```python
from build123d import *

# Parameters (mm, degrees)
ESQUISSE1_R             = 2
BOSS_EXTRU_1_DEPTH      = 3
CONG_2_R                = 10
CONG_3_R                = 10
ENL_V_MAT_EXTRU_1_DEPTH = 198.287332615
CONG_4_R                = 5


with BuildPart() as part:
    # Esquisse1 → Boss.-Extru.1 (new body)
    with BuildSketch(Plane(origin=(0, 0, 0), x_dir=(1, 0, 0), z_dir=(0, 1, 0))):
        Polygon((-150, 0), (-75, -129.903810568), (75, -129.903810568), (150, 0), (75, 129.903810568), (-75, 129.903810568), align=None)
        with Locations(Location((15.5, -109.903810568, 0), (0, 0, 270))):
            Circle(ESQUISSE1_R, mode=Mode.SUBTRACT)
        with Locations(Location((-15.5, -109.903810568, 0), (0, 0, 90))):
            Circle(ESQUISSE1_R, mode=Mode.SUBTRACT)
        with Locations(Location((15.5, -59.903810568, 0), (0, 0, 270))):
            Circle(ESQUISSE1_R, mode=Mode.SUBTRACT)
        with Locations(Location((-15.5, -59.903810568, 0), (0, 0, 90))):
            Circle(ESQUISSE1_R, mode=Mode.SUBTRACT)
        with Locations(Location((-87.429491924, -68.375299042, 0), (0, 0, 270))):
            Circle(ESQUISSE1_R, mode=Mode.SUBTRACT)
        with Locations(Location((-102.929491924, -41.528511525, 0), (0, 0, 90))):
            Circle(ESQUISSE1_R, mode=Mode.SUBTRACT)
        with Locations(Location((-59.628221735, -16.528511525, 0), (0, 0, 90))):
            Circle(ESQUISSE1_R, mode=Mode.SUBTRACT)
        with Locations(Location((-44.128221735, -43.375299042, 0), (0, 0, 270))):
            Circle(ESQUISSE1_R, mode=Mode.SUBTRACT)
        with Locations(Location((-102.929491924, 41.528511525, 0), (0, 0, 270))):
            Circle(ESQUISSE1_R, mode=Mode.SUBTRACT)
        with Locations(Location((-87.429491924, 68.375299042, 0), (0, 0, 90))):
            Circle(ESQUISSE1_R, mode=Mode.SUBTRACT)
        with Locations(Location((-44.128221735, 43.375299042, 0), (0, 0, 90))):
            Circle(ESQUISSE1_R, mode=Mode.SUBTRACT)
        with Locations(Location((-59.628221735, 16.528511525, 0), (0, 0, 270))):
            Circle(ESQUISSE1_R, mode=Mode.SUBTRACT)
        with Locations(Location((-15.5, 109.903810568, 0), (0, 0, 270))):
            Circle(ESQUISSE1_R, mode=Mode.SUBTRACT)
        with Locations(Location((15.5, 109.903810568, 0), (0, 0, 90))):
            Circle(ESQUISSE1_R, mode=Mode.SUBTRACT)
        with Locations(Location((15.5, 59.903810568, 0), (0, 0, 90))):
            Circle(ESQUISSE1_R, mode=Mode.SUBTRACT)
        with Locations(Location((-15.5, 59.903810568, 0), (0, 0, 270))):
            Circle(ESQUISSE1_R, mode=Mode.SUBTRACT)
        with Locations(Location((87.429491924, 68.375299042, 0), (0, 0, 270))):
            Circle(ESQUISSE1_R, mode=Mode.SUBTRACT)
        with Locations(Location((102.929491924, 41.528511525, 0), (0, 0, 90))):
            Circle(ESQUISSE1_R, mode=Mode.SUBTRACT)
        with Locations(Location((59.628221735, 16.528511525, 0), (0, 0, 90))):
            Circle(ESQUISSE1_R, mode=Mode.SUBTRACT)
        with Locations(Location((44.128221735, 43.375299042, 0), (0, 0, 270))):
            Circle(ESQUISSE1_R, mode=Mode.SUBTRACT)
        with Locations(Location((102.929491924, -41.528511525, 0), (0, 0, 270))):
            Circle(ESQUISSE1_R, mode=Mode.SUBTRACT)
        with Locations(Location((87.429491924, -68.375299042, 0), (0, 0, 90))):
            Circle(ESQUISSE1_R, mode=Mode.SUBTRACT)
        with Locations(Location((44.128221735, -43.375299042, 0), (0, 0, 90))):
            Circle(ESQUISSE1_R, mode=Mode.SUBTRACT)
        with Locations(Location((59.628221735, -16.528511525, 0), (0, 0, 270))):
            Circle(ESQUISSE1_R, mode=Mode.SUBTRACT)
    extrude(amount=BOSS_EXTRU_1_DEPTH)

    # Congé2
    cong_2_edges = [part.edges().sort_by_distance(p)[0] for p in [
        (-75, 1.5, -129.903810568),
    ]]
    fillet(cong_2_edges, radius=CONG_2_R)

    # Congé3
    cong_3_edges = [part.edges().sort_by_distance(p)[0] for p in [
        (75, 1.5, -129.903810568),
        (150, 1.5, 0),
        (75, 1.5, 129.903810568),
        (-75, 1.5, 129.903810568),
        (-150, 1.5, 0),
    ]]
    fillet(cong_3_edges, radius=CONG_3_R)

    # Esquisse3 → Enlèv. mat.-Extru.1 (cut, through all)
    with BuildSketch(Plane(origin=(0, 3, 0), x_dir=(1, 0, 0), z_dir=(0, 1, 0))):
        with BuildLine():
            Line((-69.226497308, -129.903810568), (-29.814110868, -129.903810568))
            Line((-29.814110868, -129.903810568), (-29.814110868, -51.639554805))
            Line((-29.814110868, -51.639554805), (-97.592944566, -90.771682686))
            Line((-97.592944566, -90.771682686), (-77.886751346, -124.903810568))
            ThreePointArc((-77.886751346, -124.903810568), (-74.226497308, -128.564064606), (-69.226497308, -129.903810568))
        make_face()
        with BuildLine():
            Line((-147.113248654, -5), (-127.5737221, -38.843452747))
            Line((-127.5737221, -38.843452747), (-59.794888402, 0.288675135))
            Line((-59.794888402, 0.288675135), (-127.0737221, 39.132127881))
            Line((-127.0737221, 39.132127881), (-127.3237221, 39.276465449))
            Line((-127.3237221, 39.276465449), (-147.113248654, 5))
            ThreePointArc((-147.113248654, 5), (-148.452994616, 0), (-147.113248654, -5))
        make_face()
        with BuildLine():
            Line((-77.886751346, 124.903810568), (-97.592944566, 90.771682686))
            Line((-97.592944566, 90.771682686), (-97.092944566, 90.483007552))
            Line((-97.092944566, 90.483007552), (-29.814110868, 51.639554805))
            Line((-29.814110868, 51.639554805), (-29.814110868, 129.903810568))
            Line((-29.814110868, 129.903810568), (-69.226497308, 129.903810568))
            ThreePointArc((-69.226497308, 129.903810568), (-74.226497308, 128.564064606), (-77.886751346, 124.903810568))
        make_face()
        with BuildLine():
            Line((30.147444201, 51.639554805), (97.6762779, 90.627345119))
            Line((97.6762779, 90.627345119), (77.886751346, 124.903810568))
            ThreePointArc((77.886751346, 124.903810568), (74.226497308, 128.564064606), (69.226497308, 129.903810568))
            Line((69.226497308, 129.903810568), (30.147444201, 129.903810568))
            Line((30.147444201, 129.903810568), (30.147444201, 129.326460298))
            Line((30.147444201, 129.326460298), (30.147444201, 51.639554805))
        make_face()
        with BuildLine():
            Line((60.128221735, -0.288675135), (127.407055434, -39.132127881))
            Line((127.407055434, -39.132127881), (147.113248654, -5))
            ThreePointArc((147.113248654, -5), (148.452994616, 0), (147.113248654, 5))
            Line((147.113248654, 5), (127.407055434, 39.132127881))
            Line((127.407055434, 39.132127881), (59.628221735, 0))
            Line((59.628221735, 0), (60.128221735, -0.288675135))
        make_face()
        with BuildLine():
            Line((29.647444201, -51.92822994), (29.647444201, -129.903810568))
            Line((29.647444201, -129.903810568), (69.226497308, -129.903810568))
            ThreePointArc((69.226497308, -129.903810568), (74.226497308, -128.564064606), (77.886751346, -124.903810568))
            Line((77.886751346, -124.903810568), (97.4262779, -91.060357821))
            Line((97.4262779, -91.060357821), (29.647444201, -51.92822994))
        make_face()
        with BuildLine():
            Line((-32.564110868, -20.388611416), (-32.564110868, 22.986687627))
            ThreePointArc((-32.564110868, 22.986687627), (-37.564110868, 27.986687627), (-42.564110868, 22.986687627))
            Line((-42.564110868, 22.986687627), (-42.564110868, -20.388611416))
            ThreePointArc((-42.564110868, -20.388611416), (-37.564110868, -25.388611416), (-32.564110868, -20.388611416))
        make_face()
        with BuildLine():
            Line((33.939110868, -16.708003449), (-3.625, -38.395652971))
            ThreePointArc((-3.625, -38.395652971), (-5.455127019, -45.22577999), (1.375, -47.055907009))
            Line((1.375, -47.055907009), (38.939110868, -25.368257487))
            ThreePointArc((38.939110868, -25.368257487), (40.769237886, -18.538130468), (33.939110868, -16.708003449))
        make_face()
        with BuildLine():
            Line((-2.5, 39.045172024), (35.064110868, 17.357522502))
            ThreePointArc((35.064110868, 17.357522502), (41.894237886, 19.187649521), (40.064110868, 26.01777654))
            Line((40.064110868, 26.01777654), (2.5, 47.705426061))
            ThreePointArc((2.5, 47.705426061), (-4.330127019, 45.875299042), (-2.5, 39.045172024))
        make_face()
    extrude(amount=-ENL_V_MAT_EXTRU_1_DEPTH, mode=Mode.SUBTRACT)

    # Congé4
    cong_4_edges = [part.edges().sort_by_distance(p)[0] for p in [
        (-127.5737221, 1.5, 38.843452747),
        (-127.3237221, 1.5, -39.276465449),
        (-59.794888402, 1.5, -0.288675135),
        (-97.592944566, 1.5, -90.771682686),
        (-29.814110868, 1.5, -129.903810568),
        (-29.814110868, 1.5, -51.639554805),
        (30.147444201, 1.5, -129.903810568),
        (97.6762779, 1.5, -90.627345119),
        (30.147444201, 1.5, -51.639554805),
        (127.407055434, 1.5, -39.132127881),
        (127.407055434, 1.5, 39.132127881),
        (59.628221735, 1.5, 0),
        (97.4262779, 1.5, 91.060357821),
        (29.647444201, 1.5, 129.903810568),
        (29.647444201, 1.5, 51.92822994),
        (-29.814110868, 1.5, 51.639554805),
        (-29.814110868, 1.5, 129.903810568),
        (-97.592944566, 1.5, 90.771682686),
    ]]
    fillet(cong_4_edges, radius=CONG_4_R)


solid = part.part
```
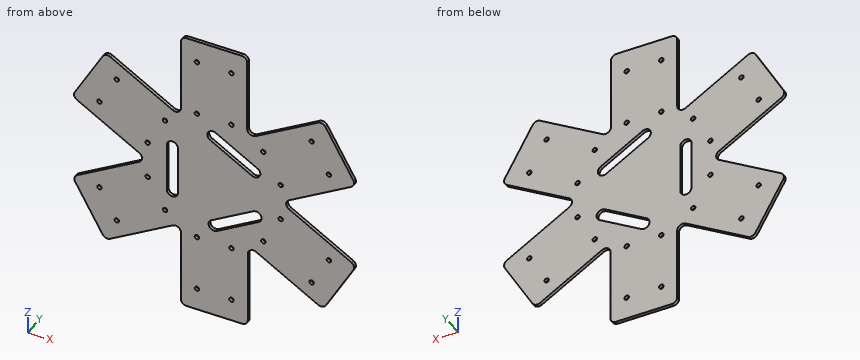
Geometry: final body of the model. Coordinates: model frame, mm. Give positions to 0.01 mm unless a question says otherwise; leave off trailing zeros. Loops run counter-clockwise (first coordinate to the right, second up) from the corner with the lowest first, then second, coordinate; pieces in that order, holes last. Notation, with made-up numbers: (0, 36.5) - (37, 36.5) arc R13 cw to (37, 50.5) - close; hole circle Ø10 at (24, -20). An arc over 180 degrees is marked (long way). Answer as CSV lines item,"result". Start each with the question number.
(1) Ray query, line 1 along Z through (x, y) = (-15, 2.7); line 2 along Z through (x, y) = (32.5, 0.3); line 3 along Z through (x, y) = (-103.5, 2.35). Return the intervals inside material, ascending. Write a range as [from, to].
(2) Pin query (flat end, axial travel): P1, Ø0.9, axis at y = 2, z = -10, coming from the +X side; P2, Ø1, axis at y = 1.5, z = 65, coming from the +X side; P3, Ø3.5, axis at x = 15.5, z = 59.9, coming from the -Y side; P4, Ø1, axis at y = 1, z = -88, coming from the +X side. Return the tip coordinate at first contact, or that it passes through.
(3) Section query C-C (z = 104). Output: boundary loops of the cut face in (x, y).
(4) Section query A-A (z = -33.5). Output: boundary loops of the cut face in (x, y).
(5) Section query D-D (z = 9). Output: boundary loops of the cut face in (x, y), and give its area (3 significant figures).
(6) Section query B-B (x = 7). Output: boundary loops of the cut face in (y, z), and give its area (3 significant figures).
Worked answers:
1,line 1,"z = [-129.9, -111.84], [-107.97, -61.84], [-57.97, 57.97], [61.84, 107.97], [111.84, 129.9]"
1,line 2,"z = [-56.06, -30.38], [-18.84, 17.54], [29.09, 56.07]"
1,line 3,"z = [-80.54, -43.45], [-39.61, -25.52], [24.94, 39.61], [43.45, 80.54]"
2,P1,"stops at x = 77.73"
2,P2,"stops at x = 112.76"
2,P3,"passes through"
2,P4,"stops at x = 99.21"
3,outline,"(-29.81, 0) - (29.65, 0) - (29.65, 3) - (-29.81, 3) - close"
4,outline,"(-117.32, 0) - (7.1, 0) - (7.1, 3) - (-117.32, 3) - close; (27.1, 0) - (117.65, 0) - (117.65, 3) - (27.1, 3) - close"
5,outline,"(-75.88, 0) - (-42.56, 0) - (-42.56, 3) - (-75.88, 3) - close; (-32.56, 0) - (75.22, 0) - (75.22, 3) - (-32.56, 3) - close"
5,area,"423 mm^2"
6,outline,"(0, -129.9) - (3, -129.9) - (3, -45.11) - (0, -45.11) - close; (0, -33.56) - (3, -33.56) - (3, 32.26) - (0, 32.26) - close; (0, 43.81) - (3, 43.81) - (3, 129.9) - (0, 129.9) - close"
6,area,"710 mm^2"
